```python
from build123d import *

# Parameters (mm, degrees)
SKETCH1_W           = 62.6
SKETCH1_H           = 72.6
BOSS_EXTRUDE1_DEPTH = 24.14
SKETCH2_W           = 50
SKETCH2_H           = 24
BOSS_EXTRUDE2_DEPTH = 19
SKETCH3_W           = 62.6
SKETCH3_H           = 72.6
BOSS_EXTRUDE3_DEPTH = 7.3
FILLET1_R           = 2
FILLET2_R           = 11


with BuildPart() as part:
    # Sketch1 → Boss-Extrude1 (new body)
    with BuildSketch(Plane(origin=(0, 0, 0), x_dir=(1, 0, 0), z_dir=(0, 1, 0))):
        Rectangle(SKETCH1_W, SKETCH1_H)
    extrude(amount=BOSS_EXTRUDE1_DEPTH)

    # Sketch2 → Boss-Extrude2 (add)
    with BuildSketch(Plane.XZ):
        with Locations((0, -17.2)):
            Rectangle(SKETCH2_W, SKETCH2_H)
    extrude(amount=BOSS_EXTRUDE2_DEPTH)

    # Sketch3 → Boss-Extrude3 (add)
    with BuildSketch(Plane(origin=(0, 24.14, 0), x_dir=(1, 0, 0), z_dir=(0, 1, 0))):
        Rectangle(SKETCH3_W, SKETCH3_H)
    extrude(amount=BOSS_EXTRUDE3_DEPTH)

    # Fillet1
    fillet1_edges = [part.edges().sort_by_distance(p)[0] for p in [
        (0, 31.44, 36.3),
        (31.3, 31.44, 0),
        (0, 31.44, -36.3),
        (-31.3, 31.44, 0),
        (0, 0, 36.3),
        (-31.3, 0, 0),
        (0, 0, -36.3),
        (31.3, 0, 0),
        (31.3, 15.72, 36.3),
        (-31.3, 15.72, 36.3),
        (-31.3, 15.72, -36.3),
        (31.3, 15.72, -36.3),
    ]]
    fillet(fillet1_edges, radius=FILLET1_R)

    # Fillet2
    fillet2_edges = [part.edges().sort_by_distance(p)[0] for p in [
        (-25, -9.5, -5.2),
        (-25, -9.5, -29.2),
        (25, -9.5, -29.2),
        (25, -9.5, -5.2),
    ]]
    fillet(fillet2_edges, radius=FILLET2_R)


solid = part.part
```
Could you check a few things on this model? Use its own coordinates, in mm. A direction names the side the tool comes from. Coordinates: 2 decimals unless noted, no trailing zeros. Write each loop counter-clockwise with the first axis right and the second up, starting at its lowest first coordinate (ties: lowest second). Pieces come first, ordered by that corner, then holes. Notation, with made-up numbers: (-28, 27) -> (-18, 27) arc R27 ccw to (-18, 49) -> close; hole circle Ø2 at (54, -0.5). An arc over 180 degrees is marked (long way). Write item = value, one per line. Start each with the question number.
(1) I want a section at B-B (z = 25.5). Please give me the cut outline in (x, y), plus the area to 3 significant figures.
(2) I want a section at C-C (x = 8). Please give me the cut outline in (y, z).
(3) I want a section at D-D (x = -23). Please give me the cut outline in (y, z), plus the area to 3 significant figures.
(4) I want a section at A-A (y = -7). Please give me the cut outline in (x, z).
(5) Will these pins go through, and if not, where does the flat tip stop? pin 1 (5 mm diameter, centred on y = -13, z = -9, fed in from +X); pin 2 (0.6 mm diameter, centred on y = -13.5, z = -17, fed in from +X); pin 3 (5.5 mm diameter, centred on x = -0.5, y = -9.5, fed in from +Z).
(6) I need wall thicknesses on line 1 (Y direction, x = -7.5, z = 22); line 2 (Z direction, x = 1, y = -5.5); line 3 (X direction, y = -1, z = -16.5). Which ranges of each line are inside material? Lowest first, please. Write a range as [from, to].
(7) Which directions (+Z, -Z, +X, -X, +Y, -Y) give clear straight access to the entire face, cutting with the end or side of a thin tool? Please do faces 1 (the face through (-21.863, -9.633, -8.508)), 2 (the face through (21.863, -9.633, -25.892)), 3 (the face through (0, -9, -5.2)).
Result set:
q1.outline = (-31.3, 2) arc R2 ccw to (-29.3, 0) -> (29.3, 0) arc R2 ccw to (31.3, 2) -> (31.3, 29.44) arc R2 ccw to (29.3, 31.44) -> (-29.3, 31.44) arc R2 ccw to (-31.3, 29.44) -> close
q1.area = 1,960 mm2
q2.outline = (-19, -29.2) -> (0, -29.2) -> (0, -34.3) arc R2 ccw to (2, -36.3) -> (29.44, -36.3) arc R2 ccw to (31.44, -34.3) -> (31.44, 34.3) arc R2 ccw to (29.44, 36.3) -> (2, 36.3) arc R2 ccw to (0, 34.3) -> (0, -5.2) -> (-19, -5.2) -> close
q3.outline = (-19, -24.52) -> (0, -24.52) -> (0, -34.3) arc R2 ccw to (2, -36.3) -> (29.44, -36.3) arc R2 ccw to (31.44, -34.3) -> (31.44, 34.3) arc R2 ccw to (29.44, 36.3) -> (2, 36.3) arc R2 ccw to (0, 34.3) -> (0, -9.88) -> (-19, -9.88) -> close
q3.area = 2,560 mm2
q4.outline = (-25, -18.2) arc R11 ccw to (-14, -29.2) -> (14, -29.2) arc R11 ccw to (25, -18.2) -> (25, -16.2) arc R11 ccw to (14, -5.2) -> (-14, -5.2) arc R11 ccw to (-25, -16.2) -> close
q5.pin_1 = 23.95
q5.pin_2 = 25
q5.pin_3 = -5.2
q6.line_1 = [0, 31.44]
q6.line_2 = [-29.2, -5.2]
q6.line_3 = [-25, 25]
q7.face_1 = +Z, -X, -Y
q7.face_2 = -Z, +X, -Y
q7.face_3 = +Z, +X, -X, -Y
